Design review of the part shown in the three views and the two pictorial views. Dimensions are in mm from the part's minimum x, y and z. A direction names the side the tool comes from. Coordinates: 2 decimals unless noted, no trailing zeros. Write each loop counter-clockwise with the first axis right and the second up, starting at its lowest first coordinate (ties: lowest second). Pieces come first, ordered by that corner, then holes. Notation, with made-up numbers: (81, -15) - (93, -15) arc R29 cw to (93, 13) - close; hole circle Ø8 at (31.5, 44). An arc over 180 degrees is marked (long way). Write each question's results on one line, items separated by ' | '.
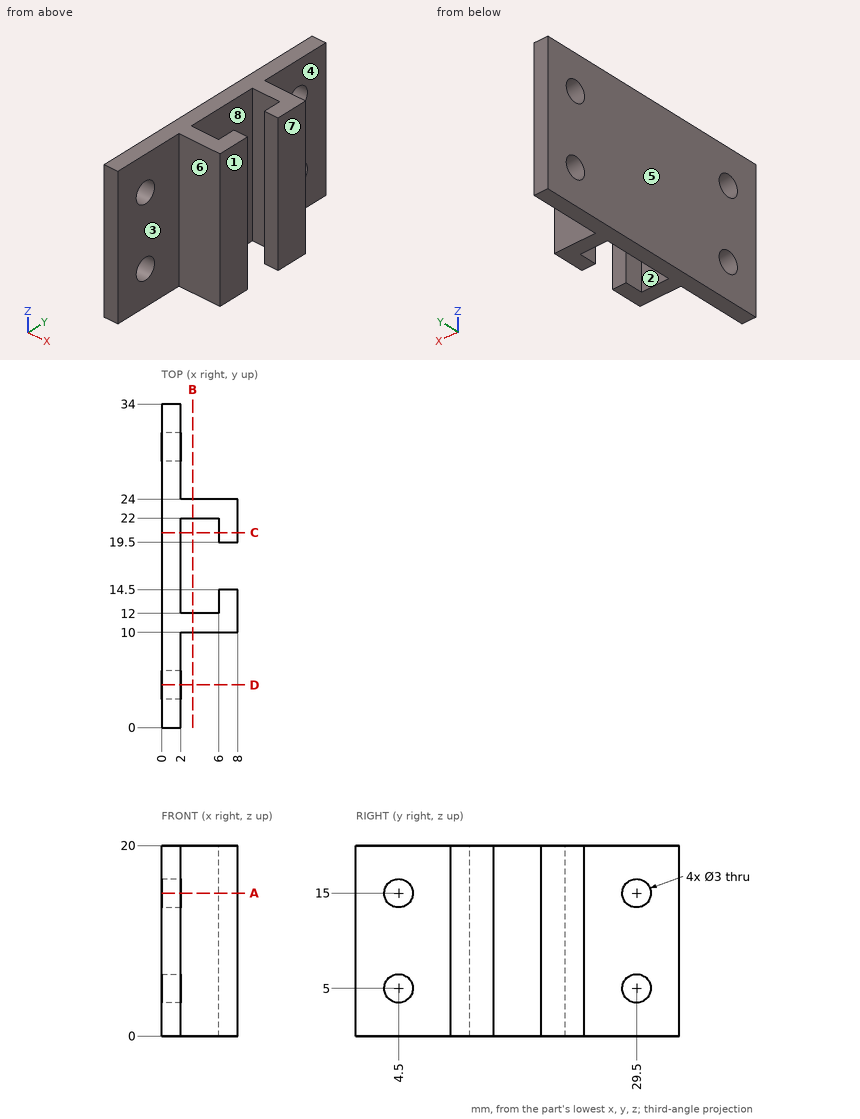
Q1. For pin 1 (1.8 mm diameter, centred on x = 5.5, z = 14.5, fed in from +Y); pin 2 (8 mm diameter, centred on y = 30.5, z = 9.5, fed in from +X); pin 3 (1.6 mm diameter, centred on x = 7, z = 10, fed in from -Y), all flat-tipped, find the tip position at first contact; note any pin that passes through.
Results found:
pin 1: y = 24 | pin 2: x = 2 | pin 3: y = 10
Q2. Take a section at B-B on x = 3.25. State the section outline as (y, z) points.
Results found:
outline: (10, 0) - (12, 0) - (12, 20) - (10, 20) - close; (22, 0) - (24, 0) - (24, 20) - (22, 20) - close
Q3. For the marked faces 1, 2, 3, 4 and 5, list the 3-axis set-ups (+Z, -Z, +X, -X, +Y, -Y) from which the entire face can be reached by the end or side of a thin tool; tool diameter is ignored.
Results found:
face 1: +Z, -Z, +X, +Y, -Y | face 2: +Z, -Z | face 3: +Z, -Z, +X, -Y | face 4: +Z, -Z, +X, +Y | face 5: +Z, -Z, -X, +Y, -Y
Q4. Take a section at D-D on y = 4.5. State the section outline as (x, z) points, plus the area to 3 significant figures.
Results found:
outline: (0, 0) - (2, 0) - (2, 3.5) - (0, 3.5) - close; (0, 6.5) - (2, 6.5) - (2, 13.5) - (0, 13.5) - close; (0, 16.5) - (2, 16.5) - (2, 20) - (0, 20) - close | area: 28.0 mm2
Q5. Take a section at C-C on y = 20.5. State the section outline as (x, z) points, plus the area to 3 significant figures.
Results found:
outline: (0, 0) - (2, 0) - (2, 20) - (0, 20) - close; (6, 0) - (8, 0) - (8, 20) - (6, 20) - close | area: 80.0 mm2
Q6. Take a section at A-A on z = 15. State the section outline as (x, y) points.
Results found:
outline: (0, 0) - (2, 0) - (2, 3) - (0, 3) - close; (0, 6) - (2, 6) - (2, 10) - (8, 10) - (8, 14.5) - (6, 14.5) - (6, 12) - (2, 12) - (2, 22) - (6, 22) - (6, 19.5) - (8, 19.5) - (8, 24) - (2, 24) - (2, 28) - (0, 28) - close; (0, 31) - (2, 31) - (2, 34) - (0, 34) - close
Q7. Wall thickness on line 1 along Y through (x, z) = (0.8, 5); line 2 along X through (y, z) = (12.5, 7.5); line 3 along Y through (x, z) = (6.5, 15): over which ranges is each line inside the solid? List them lowest first. Write a range as from..to.
Results found:
line 1: 0..3, 6..28, 31..34 | line 2: 0..2, 6..8 | line 3: 10..14.5, 19.5..24
Q8. Mouldability with a two-part tool opening along Y and no side actions: class the marked faces 6, 7 and 8 as pulls with the +Y half, pulls with the -Y half, needs draft (parallel to the pull), parting line crosses it, or undercut.
Results found:
face 6: pulls with the -Y half | face 7: needs draft | face 8: undercut
